Input: part model. Units: mm. Frame: model coordinates. A direction names the side the tool comes from. Round coordinates to 2 decimals unless told otherwise and drop trailing zeros. Loops run counter-clockwise (first coordinate to the right, second up) from the corner with the lowest first, then second, coordinate; pieces in that order, holes last. Notation, with made-up numbers: (-6.5, -34) -> (24.5, -34) arc R23 ccw to (24.5, 2) -> close; hole circle Ø10 at (70, 67.25). An arc over 180 degrees is marked (long way). Answer as a JSON object with one key per item and string values.
Autodesk Inventor part; units mm, degrees
ref_plane "YZ Plane" through (0, 0, 0) normal (1, 0, 0) x (0, 1, 0)
ref_plane "XZ Plane" through (0, 0, 0) normal (0, 1, 0) x (-1, 0, 0)
ref_plane "XY Plane" through (0, 0, 0) normal (0, 0, 1) x (1, 0, 0)
sketch "Esboço1" plane through (0, 0, 0) normal (0, 0, 1) x (1, 0, 0)
  circle A0 centre (8.001, 0) radius 2.4
  circle A1 centre (8.001, 0) radius 2.4
  circle A2 centre (64.001, 0) radius 2.4
  circle A3 centre (64.001, 0) radius 2.4
  line L0 (58.601, 8.5) -> (13.401, 8.5)
  line L1 (58.601, -12.1) -> (58.601, 8.5)
  line L2 (13.401, 8.5) -> (13.401, -12.1)
  line L3 (67.806, 3.9) -> (60.196, 3.9)
  arc A4 (60.101, 0) -> (67.901, 0) centre (64.001, 0) ccw
  line L4 (60.101, 0) -> (60.101, 8.5)
  line L5 (60.101, 8.5) -> (11.901, 8.5)
  arc A5 (4.101, 0) -> (11.901, 0) centre (8.001, 0) ccw
  line L6 (11.901, 0) -> (11.901, 8.5)
  line L7 (4.101, 0) -> (4.101, 8.5)
  line L8 (4.101, 8.5) -> (4.101, 10.5)
  line L9 (67.901, 0) -> (67.901, 10.2879)
  line L10 (67.901, 10.5) -> (4.101, 10.5)
  line L11 (67.901, 10.1485) -> (67.901, 10.5)
  point P0 (0, 0)
  dimension "d0" = 7.8
  dimension "d1" = 2
extrude "Extrusão1" add sketch "Esboço1" along normal blind 8
sketch "Esboço3" plane through (0, 0, 8) normal (0, 0, 1) x (1, 0, 0)
  circle A0 centre (23.201, -1.8) radius 7.95
  circle A1 centre (48.801, -1.8) radius 7.95
  arc A2 (60.101, 0) -> (67.901, 0) centre (64.001, 0) ccw
  line L0 (11, -1.8) -> (11, 9)
  line L1 (11, 9) -> (60.5412, 9)
  line L2 (60.5412, 9) -> (60.5412, -1.8)
  line L3 (15.251, -1.8) -> (11, -1.8)
  line L4 (60.5412, -1.8) -> (56.751, -1.8)
  line L5 (40.851, -1.8) -> (31.151, -1.8)
  point P0 (0, 0)
extrude "Extrusão2" add sketch "Esboço3" against normal blind 2 contours A0 L3 L0 L1 L2 L4 A1 L5
sketch "Esboço4" plane through (0, 0, 8) normal (0, 0, 1) x (1, 0, 0)
  circle A0 centre (8, 0) radius 3.1
  circle A1 centre (64.001, 0) radius 2.4
  circle A2 centre (64, 0) radius 3.1
  circle A3 centre (8.001, 0) radius 2.4
  point P0 (0, 0)
  dimension "d6" = 6.2
  dimension "d7" = 6.2
extrude "Extrusão3" cut sketch "Esboço4" against normal blind 1
sketch "Esboço5" plane through (0, 0, 0) normal (0, 0, -1) x (-1, 0, 0)
  circle A0 centre (-8, 0) radius 3.1
  circle A1 centre (-8.001, 0) radius 2.4
  circle A2 centre (-64.001, 0) radius 2.4
  circle A3 centre (-64.001, 0) radius 3.1
  point P0 (0, 0)
  dimension "d10" = 6.2
extrude "Extrusão4" cut sketch "Esboço5" against normal blind 1
sketch "Esboço6" plane through (0, 0, 8) normal (0, 0, 1) x (1, 0, 0)
  line L0 (33.501, 12.5) -> (33.501, 15)
  line L1 (38.501, 15) -> (38.501, 12.5)
  line L2 (4.101, 10.5) -> (4.101, 0)
  line L3 (-3.999, -3.9) -> (-3.999, 3.9)
  circle A0 centre (36.001, 15) radius 1
  circle A1 centre (36.001, 15) radius 2.5
  arc A2 (31.501, 10.5) -> (33.501, 12.5) centre (31.501, 12.5) ccw
  arc A3 (38.501, 12.5) -> (40.501, 10.5) centre (40.501, 12.5) ccw
  line L4 (40.501, 10.5) -> (31.501, 10.5)
  line L5 (67.901, 10.5) -> (4.101, 10.5)
  point P0 (0, 0)
  dimension "d19" = 29.4
  dimension "d20" = 2
  dimension "d22" = 2
  dimension "d23" = 2
extrude "Extrusão5" add sketch "Esboço6" against normal blind 2
sketch "Esboço8" plane through (0, 0, 0) normal (0, 0, -1) x (-1, 0, 0)
  line L0 (-28.001, 3.9) -> (-28.001, 3.6)
  line L1 (-11.901, 8.5) -> (-60.101, 8.5)
  line L2 (-67.901, 10.5) -> (-4.101, 10.5)
  line L3 (-28.001, 8.5) -> (-44.001, 8.5)
  line L4 (-44.001, 8.5) -> (-44.001, 10.5)
  line L5 (-44.001, 10.5) -> (-28.001, 10.5)
  line L6 (-28.001, 10.5) -> (-28.001, 8.5)
  point P0 (0, 0)
  dimension "d24" = 16
extrude "Extrusão6" add sketch "Esboço8" along normal blind 8
sketch "Esboço9" plane through (11.901, 8.5, 6) normal (0, -1, 0) x (1, 0, 0)
  circle A0 centre (28.1, -10) radius 2.4
  circle A1 centre (20.1, -10) radius 2.4
  arc A2 (16.1, -10) -> (20.1, -14) centre (20.1, -10) ccw
  line L0 (32.1, -14) -> (16.1, -14)
  arc A3 (28.1, -14) -> (32.1, -10) centre (28.1, -10) ccw
  line L1 (32.1, -6) -> (32.1, -14)
  line L2 (16.1, -10) -> (16.1, -14)
  line L3 (32.1, -14) -> (32.1, -10)
  line L4 (16.1, -14) -> (20.1, -14)
  line L5 (28.1, -14) -> (32.1, -14)
  point P0 (-11.901, -6)
  point P1 (28.1, -14)
extrude "Extrusão7" cut sketch "Esboço9" against normal blind 6.75
sketch "Esboço10" plane through (64.001, 0, 1) normal (0, 0, -1) x (-1, 0, 0)
  circle A0 centre (0, 0) radius 2.4
  circle A1 centre (56, 0) radius 2.4
  circle A2 centre (0, 0) radius 2.5
  circle A3 centre (56, 0) radius 2.5
  point P0 (64.001, 0)
  dimension "d29" = 5
  dimension "d30" = 5
extrude "Extrusão8" cut sketch "Esboço10" against normal blind 15.25
sketch "Esboço11" plane through (4.101, 10.5, 8) normal (0, 1, 0) x (1, 0, 0)
  circle A0 centre (27.9, 12) radius 2.4
  circle A1 centre (35.9, 12) radius 2.4
  circle A2 centre (27.9, 12) radius 2.5
  circle A3 centre (35.9, 12) radius 2.5
  point P0 (-4.101, 8)
  dimension "d33" = 5
  dimension "d34" = 5
extrude "Extrusão9" cut sketch "Esboço11" against normal blind 10
properties part number "apoio ultrassonico"
1) Draft query along Z for faces 1 (the face through (60.101, 4, 3)), 2 (the face through (36, 7, 8)), 3 (the face through (36, 10, -8)), 4 (the face through (34.386, 9.514, -4.751)). Return one class per face: +Z half, -Z half, draft (parallel to the pull), parting line (faces both ways), or undercut.
Output:
{"face 1": "draft", "face 2": "+Z half", "face 3": "-Z half", "face 4": "undercut"}
2) Section B-B, the plane x = 8. Output: boundary loops of the cut face in (y, z).
Output:
{"outline": "(-3.9, 0) -> (-3.1, 0) -> (-3.1, 1) -> (-2.5, 1) -> (-2.5, 7) -> (-3.1, 7) -> (-3.1, 8) -> (-3.9, 8) -> close; (2.5, 1) -> (3.1, 1) -> (3.1, 0) -> (10.5, 0) -> (10.5, 8) -> (3.1, 8) -> (3.1, 7) -> (2.5, 7) -> close"}
3) Section D-D, the plane z = -0.75. Output: boundary loops of the cut face in (x, y), plus the area to 3 significant figures.
Output:
{"outline": "(28, 8.5) -> (44, 8.5) -> (44, 10.5) -> (28, 10.5) -> close", "area": "32.0 mm^2"}
4) Section A-A, the plane z = 3.75. Output: boundary loops of the cut face in (x, y).
Output:
{"outline": "(4.1, 0) arc R3.9 ccw to (11.9, 0) -> (11.9, 8.5) -> (60.1, 8.5) -> (60.1, 0) arc R3.9 ccw to (67.9, 0) -> (67.9, 10.5) -> (4.1, 10.5) -> close; hole circle Ø5 at (8, 0); hole circle Ø5 at (64, 0)"}
5) Contact query for flat-ended pins moving along their axis: P1, Ø5, axis at x = 22, z = -1.5, coming from the +Y side; P2, Ø12, axis at x = 59.5, y = 2.5, coming from the -Z side; P3, Ø1.6, axis at x = 58, z = 6.5, coming from the -Y side. Output: stop coordinate, or through.
Output:
{"P1": "stops at y = 10.5", "P2": "stops at z = 0", "P3": "stops at y = -1.8"}
6) Section C-C, the plane y = 3.75. Output: boundary loops of the cut face in (x, z).
Output:
{"outline": "(4.1, 0) -> (11.9, 0) -> (11.9, 6) -> (17.51, 6) -> (17.51, 8) -> (4.1, 8) -> close; (28.89, 6) -> (43.11, 6) -> (43.11, 8) -> (28.89, 8) -> close; (54.49, 6) -> (60.1, 6) -> (60.1, 0) -> (67.9, 0) -> (67.9, 8) -> (54.49, 8) -> close"}
7) Reachability of faces 5 (the face through (11.6, 6, 0)), 6 (the face through (36, 13, 6)), 7 (the face through (38.501, 14, 7)), 8 (the face through (13, -1.8, 7)), 9 (the face through (32.9, 11.07, 7.01)) from +Z, -Z, +X, -X, +Y, -Y: full face, straight path, thin tool, end or side. Return the list, or none.
Output:
{"face 5": "-Z, -X, +Y, -Y", "face 6": "-Z, +X, -X, +Y", "face 7": "+Z, -Z, +X, +Y", "face 8": "+Z, -Z, -Y", "face 9": "+Z, -Z, -X, +Y"}
8) Ray query, probe 1 along X at (y, z) = (9.15, -4); probe 2 along Y at (x, z) = (47, 1.5); probe 3 along Y at (x, z) = (15, 7). Return the intervals inside material, ascending.
Output:
{"probe 1": "x = 28 to 29.5, 34.5 to 37.5, 42.5 to 44", "probe 2": "y = 8.5 to 10.5", "probe 3": "y = -1.8 to 10.5"}
